Model file for the job. Use its own axes, mm. Face numbers are marked on the shaded views. A direction names the side the tool comes from. Round coordinates to 2 decimals unless told otherwise and drop trailing zeros. Order: outer loops, then holes, each group sorted by start corner. A loop starts at its lowest first (then second) coordinate and runs counter-clockwise, first axis right, second up. Notation, with made-up numbers: (3.5, 43.25) -> (60.5, 43.25) arc R20 cw to (60.5, 72.25) -> close; hole circle Ø2 at (63.5, -24.5). An arc over 180 degrees is marked (long way). Answer as CSV lines item,"result".
```python
from build123d import *

# Parameters (mm, degrees)
SKICA1_W                    = 69
SKICA1_H                    = 52
SKICA1_W_2                  = 65
SKICA1_H_2                  = 48
VYSUNOUT_TENKOST_NN_1_DEPTH = 23
SKICA2_W                    = 10
SKICA2_H                    = 2
SKICA2_W_2                  = 2
SKICA2_H_2                  = 12
P_IDAT_EBRA_DEPTH           = 23
SKICA3_W                    = 2
SKICA3_H                    = 6
SKICA3_W_2                  = 12
SKICA3_H_2                  = 2
ODEBRAT_8_MM_DEPTH          = 8
SKICA4_W                    = 8.43
SKICA4_H                    = 2
SKICA4_W_2                  = 7.795
ODEBRAT_7_MM_DEPTH          = 7
ODEBRAT_3_5_MM_DEPTH        = 3.5
SKICA6_W                    = 51.7
SKICA6_H                    = 42.1
ODEBRAT_2_MM_DEPTH          = 2
SKICA8_W                    = 69
SKICA8_H                    = 52
P_IDAT_DNO_DEPTH            = 1
SKICA9_W                    = 2
SKICA9_H                    = 21
SKICA9_W_2                  = 65
SKICA9_H_2                  = 2
P_IDAT_EBRA_DNO_DEPTH       = 2
SKICA10_W                   = 9
SKICA10_H                   = 12
ODEBRAT_VYP_NA_DEPTH        = 24
P_IDAT_H_EK_DEPTH           = 2
SKICA12_W                   = 3
SKICA12_H                   = 3
ODEBRAT_VYSUNUT_M1_DEPTH    = 24.5
SKICA13_W                   = 3
SKICA13_H                   = 3
ODEBRAT_VYSUNUT_M2_DEPTH    = 24.5
ODEBRAT_VYSUNUT_M3_REACH    = 54
SKICA14_W                   = 2
SKICA14_H                   = 2
ODEBRAT_VYSUNUT_M4_DEPTH    = 24


with BuildPart() as part:
    # Skica1 → Vysunout tenkost_nn_1 (new body)
    with BuildSketch(Plane.XY):
        Rectangle(SKICA1_W, SKICA1_H)
        Rectangle(SKICA1_W_2, SKICA1_H_2, mode=Mode.SUBTRACT)
    extrude(amount=VYSUNOUT_TENKOST_NN_1_DEPTH)

    # Skica2 → P_idat _ebra (add)
    with BuildSketch(Plane.XY):
        Polygon((-32.5, -15), (-32.5, -14), (32.5, -14), (32.5, -15), (30.17, -15), (28.17, -19), (28.17, -24), (25.17, -24), (25.17, -19), (23.17, -15), (20.01, -15), (18.01, -19), (18.01, -24), (15.01, -24), (15.01, -19), (13.01, -15), (9.215, -15), (7.215, -19), (7.215, -24), (4.215, -24), (4.215, -19), (2.215, -15), (-2.215, -15), (-4.215, -19), (-4.215, -24), (-7.215, -24), (-7.215, -19), (-9.215, -15), (-13.01, -15), (-15.01, -19), (-15.01, -24), (-18.01, -24), (-18.01, -19), (-20.01, -15), (-23.17, -15), (-25.17, -19), (-25.17, -24), (-28.17, -24), (-28.17, -19), (-30.17, -15), align=None)
        with Locations((-27.5, 13)):
            Rectangle(SKICA2_W, SKICA2_H)
        with Locations((27.5, 13)):
            Rectangle(SKICA2_W, SKICA2_H)
        with Locations((11, 18)):
            Rectangle(SKICA2_W_2, SKICA2_H_2)
        with Locations((-11, 18)):
            Rectangle(SKICA2_W_2, SKICA2_H_2)
    extrude(amount=P_IDAT_EBRA_DEPTH)

    # Skica3 → Odebrat 8 mm (cut)
    with BuildSketch(Plane.XY.offset(23)):
        with Locations((-11, 15)):
            Rectangle(SKICA3_W, SKICA3_H)
        with Locations((0, 25)):
            Rectangle(SKICA3_W_2, SKICA3_H_2)
    extrude(amount=-ODEBRAT_8_MM_DEPTH, mode=Mode.SUBTRACT)

    # Skica4 → Odebrat 7 mm (cut)
    with BuildSketch(Plane.XY.offset(23)):
        with Locations((0, -25)):
            Rectangle(SKICA4_W, SKICA4_H)
        with Locations((11.1125, -25)):
            Rectangle(SKICA4_W_2, SKICA4_H)
        with Locations((-11.1125, -25)):
            Rectangle(SKICA4_W_2, SKICA4_H)
        Polygon((18.01, -24), (18.01, -26), (25.8, -26), (25.8, -24), (28.17, -24), (28.17, -19), (25.17, -19), (25.17, -24), align=None)
        Polygon((-18.01, -24), (-18.01, -26), (-25.8, -26), (-25.8, -24), (-28.17, -24), (-28.17, -19), (-25.17, -19), (-25.17, -24), align=None)
    extrude(amount=-ODEBRAT_7_MM_DEPTH, mode=Mode.SUBTRACT)

    # Skica5 → Odebrat 3_5 mm (cut)
    with BuildSketch(Plane.XY.offset(23)):
        Polygon((-25.9, -13), (25.9, -13), (25.9, -15), (20.01, -15), (20.01, -19), (-20.01, -19), (-20.01, -15), (-25.9, -15), align=None)
    extrude(amount=-ODEBRAT_3_5_MM_DEPTH, mode=Mode.SUBTRACT)

    # Skica6 → Odebrat 2 mm (cut)
    with BuildSketch(Plane.XY.offset(23)):
        with Locations((0, -2.95)):
            Rectangle(SKICA6_W, SKICA6_H)
        Polygon((-34.5, 26), (34.5, 26), (34.5, -26), (25.8, -26), (25.8, -25), (33.5, -25), (33.5, 25), (-33.5, 25), (-33.5, -25), (-25.8, -25), (-25.8, -26), (-34.5, -26), align=None)
    extrude(amount=-ODEBRAT_2_MM_DEPTH, mode=Mode.SUBTRACT)

    # Skica8 → P_idat dno (add)
    with BuildSketch(Plane.XY):
        Rectangle(SKICA8_W, SKICA8_H)
    extrude(amount=P_IDAT_DNO_DEPTH)

    # Skica9 → P_idat _ebra _dno (add)
    with BuildSketch(Plane.XY):
        with Locations((-11, -3.5)):
            Rectangle(SKICA9_W, SKICA9_H)
        with Locations((11, -3.5)):
            Rectangle(SKICA9_W, SKICA9_H)
        with Locations((0, 6)):
            Rectangle(SKICA9_W_2, SKICA9_H_2)
        with Locations((0, -8)):
            Rectangle(SKICA9_W_2, SKICA9_H_2)
    extrude(amount=P_IDAT_EBRA_DNO_DEPTH)

    # Skica10 → Odebrat vyp_na (cut, through all)
    with BuildSketch(Plane(origin=(0, 0, 0), x_dir=(-1, 0, 0), z_dir=(0, 0, -1))):
        with Locations((25, -1)):
            Rectangle(SKICA10_W, SKICA10_H)
    extrude(amount=-ODEBRAT_VYP_NA_DEPTH, mode=Mode.SUBTRACT)

    # Skica11 → P_idat h_ek (add)
    with BuildSketch(Plane(origin=(4.25, -4.25, 0), x_dir=(0.707106781, 0.707106781, 0), z_dir=(-0.707106781, 0.707106781, 0))):
        with BuildLine():
            Line((25.809397513, -1), (25.809397513, -11))
            Line((25.809397513, -11), (33.809397513, -11))
            Line((33.809397513, -11), (33.809397513, -9))
            ThreePointArc((33.809397513, -9), (29.566756826, -7.242640687), (27.809397513, -3))
            Line((27.809397513, -3), (27.809397513, -1))
            Line((27.809397513, -1), (25.809397513, -1))
        make_face()
    extrude(amount=-P_IDAT_H_EK_DEPTH)

    # Skica12 → Odebrat vysunut_m1 (cut)
    with BuildSketch(Plane(origin=(34.5, 0, 0), x_dir=(0, 0, -1), z_dir=(1, 0, 0))):
        with Locations((-12.5, 21.156854249)):
            Rectangle(SKICA12_W, SKICA12_H)
        with Locations((-12.5, -21.5)):
            Rectangle(SKICA12_W, SKICA12_H)
    extrude(amount=-ODEBRAT_VYSUNUT_M1_DEPTH, mode=Mode.SUBTRACT)

    # Skica13 → Odebrat vysunut_m2 (cut)
    with BuildSketch(Plane.ZY.offset(34.5)):
        with Locations((12.5, 21.156854249)):
            Rectangle(SKICA13_W, SKICA13_H)
        with Locations((12.5, -21.5)):
            Rectangle(SKICA13_W, SKICA13_H)
    extrude(amount=-ODEBRAT_VYSUNUT_M2_DEPTH, mode=Mode.SUBTRACT)

    # Skica14 → Odebrat vysunut_m3 (cut, up to next)
    with BuildSketch(Plane(origin=(0, 26, 0), x_dir=(1, 0, 0), z_dir=(0, 1, 0)), mode=Mode.PRIVATE) as odebrat_vysunut_m3_sk1:
        with Locations((5, -9)):
            Rectangle(SKICA14_W, SKICA14_H)
    odebrat_vysunut_m3_tool1 = extrude(odebrat_vysunut_m3_sk1.sketch, amount=-ODEBRAT_VYSUNUT_M3_REACH, mode=Mode.PRIVATE) & part.part
    add(odebrat_vysunut_m3_tool1.solids().sort_by_distance((5, 26, 9))[0], mode=Mode.SUBTRACT)
    # Skica14 → Odebrat vysunut_m3 (cut, up to next)
    with BuildSketch(Plane(origin=(0, 26, 0), x_dir=(1, 0, 0), z_dir=(0, 1, 0)), mode=Mode.PRIVATE) as odebrat_vysunut_m3_sk2:
        with Locations((-5, -9)):
            Rectangle(SKICA14_W, SKICA14_H)
    odebrat_vysunut_m3_tool2 = extrude(odebrat_vysunut_m3_sk2.sketch, amount=-ODEBRAT_VYSUNUT_M3_REACH, mode=Mode.PRIVATE) & part.part
    add(odebrat_vysunut_m3_tool2.solids().sort_by_distance((-5, 26, 9))[0], mode=Mode.SUBTRACT)

    # Skica15 → Odebrat vysunut_m4 (cut)
    with BuildSketch(Plane(origin=(12, 0, 0), x_dir=(0, 0, -1), z_dir=(1, 0, 0))):
        with BuildLine():
            Line((-1, 15.5), (-1, 12))
            Line((-1, 12), (-4.5, 12))
            ThreePointArc((-4.5, 12), (-3.474873734, 14.474873734), (-1, 15.5))
        make_face()
    extrude(amount=-ODEBRAT_VYSUNUT_M4_DEPTH, mode=Mode.SUBTRACT)


solid = part.part
```
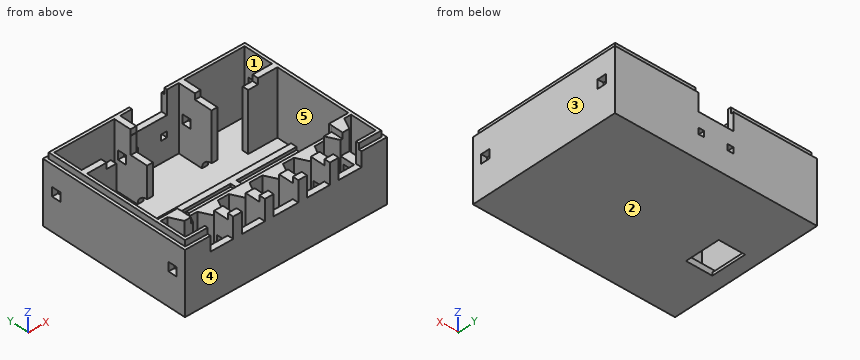
Q1. Saw through at C-C (x = 3). Write the cut outline in (y, z), plus the area to 3 significant figures.
Checks:
outline,"(-26, 0) -> (26, 0) -> (26, 15) -> (24, 15) -> (24, 1) -> (7, 1) -> (7, 2) -> (5, 2) -> (5, 1) -> (-7, 1) -> (-7, 2) -> (-9, 2) -> (-9, 1) -> (-14, 1) -> (-14, 19.5) -> (-16.57, 19.5) -> (-16.57, 1) -> (-24, 1) -> (-24, 16) -> (-26, 16) -> close"
area,"162 mm²"
Q2. Saw through at B-B (x = -16). Write the cut outline in (y, z).
Checks:
outline,"(-26, 0) -> (26, 0) -> (26, 21) -> (25, 21) -> (25, 23) -> (24, 23) -> (24, 1) -> (7, 1) -> (7, 2) -> (5, 2) -> (5, 1) -> (-7, 1) -> (-7, 2) -> (-9, 2) -> (-9, 1) -> (-14, 1) -> (-14, 19.5) -> (-19, 19.5) -> (-19, 21) -> (-24, 21) -> (-24, 23) -> (-26, 23) -> close; hole (-23, 11) -> (-20, 11) -> (-20, 14) -> (-23, 14) -> close"
Q3. Saw through at D-D (y = 11). Write the cut outline in (x, z).
Checks:
outline,"(-34.5, 0) -> (34.5, 0) -> (34.5, 21) -> (33.5, 21) -> (33.5, 23) -> (32.5, 23) -> (32.5, 1) -> (-32.5, 1) -> (-32.5, 23) -> (-33.5, 23) -> (-33.5, 21) -> (-34.5, 21) -> close"
Q4. Tool access for the marked faces 4 and 5: list every direction of +Z, -Z, +X, -X, +Y, -Y with a clear straight run to the whole face (end or side of a thin tool).
Checks:
face 4,"+Z, -Z, +X, -X, -Y"
face 5,"+Z"
Q5. Mould opens along X. For the marked faces 1, 2 and 3 say: +X half, -X half, draft (parallel to the pull), parting line (faces both ways), or undercut.
Checks:
face 1,"undercut"
face 2,"draft"
face 3,"+X half"
Q6. Wall check: L1, parallel to Y at x = -13, z = 14.5; L2, parallel to X at y = 22, z = 20.5; L3, parallel to X at y = 13.5, z = 19. Give the ranges that are in metal, low to high. Write a range as [from, to].
Checks:
L1,"[-26, -24], [-15, -14], [24, 26]"
L2,"[-34.5, -32.5], [-12, -10], [10, 12], [32.5, 34.5]"
L3,"[-34.5, -22.5], [10, 12], [22.5, 34.5]"
Q7. Flat gauge pins, fed straight in: pin 1 (5 mm diameter, centred on x = -8, y = -4.5, fed in from +Z); pin 2 (0.6 mm diameter, centred on x = -2, y = -24.5, fed in from +Z); pin 3 (1.6 mm diameter, centred on x = 24, z = 22, fed in from +Y). Where does each tip first touch, or does it go through?
Checks:
pin 1,"z = 2"
pin 2,"z = 16"
pin 3,"y = 25"
Q8. Saw through at A-A (y = -3). Write the cut outline in (x, z).
Checks:
outline,"(-34.5, 0) -> (-29.5, 0) -> (-29.5, 1) -> (-32.5, 1) -> (-32.5, 23) -> (-33.5, 23) -> (-33.5, 21) -> (-34.5, 21) -> close; (-20.5, 0) -> (34.5, 0) -> (34.5, 21) -> (33.5, 21) -> (33.5, 23) -> (32.5, 23) -> (32.5, 1) -> (12, 1) -> (12, 2) -> (10, 2) -> (10, 1) -> (-10, 1) -> (-10, 2) -> (-12, 2) -> (-12, 1) -> (-20.5, 1) -> close"
